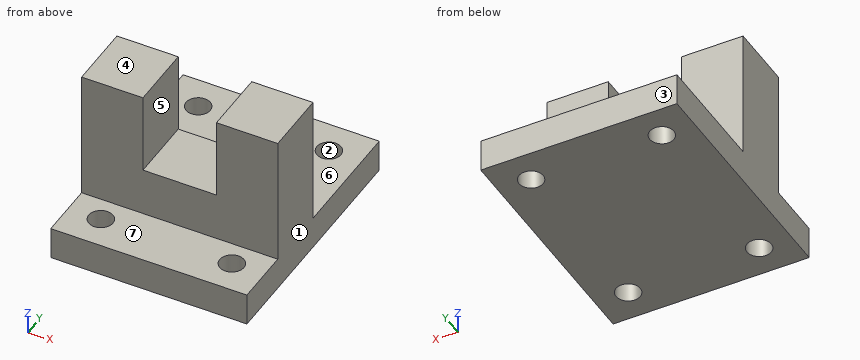
```python
from build123d import *

# Parameters (mm, degrees)
F0_W     = 23.8252
F0_H     = 31.75
F1_DEPTH = 25.4
F2_W     = 76.2
F2_H     = 12.7
F3_DEPTH = 47.625
F4_R     = 4.699
F5_DEPTH = 12.701
F6_R     = 4.699
F7_DEPTH = 33.02


with BuildPart() as f1:
    # F0 (on Front) → F1 (new body)
    with BuildSketch(Plane.XZ):
        with Locations((26.1874, 15.875)):
            Rectangle(F0_W, F0_H)
        Polygon((38.1, -31.75), (38.1, 0), (14.2748, 0), (-14.2748, 0), (-14.2748, 31.75), (-38.1, 31.75), (-38.1, -31.75), align=None)
    extrude(amount=F1_DEPTH)

    # F2 (on face) → F3 (join, symmetric)
    with BuildSketch(Plane(origin=(0, 0, 0), x_dir=(-1, 0, 0), z_dir=(0, 1, 0))):
        with Locations((0, -25.4)):
            Rectangle(F2_W, F2_H)
    extrude(amount=F3_DEPTH, both=True)

    # F4 (on face) → F5 (cut, through all)
    with BuildSketch(Plane.XY.offset(-19.05)):
        with Locations((-25.4996093811, -34.925)):
            Circle(F4_R)
        with Locations((25.4, -34.925)):
            Circle(F4_R)
    extrude(amount=-F5_DEPTH, mode=Mode.SUBTRACT)

    # F6 (on face) → F7 (cut, symmetric)
    with BuildSketch(Plane.XY.offset(-19.05)):
        with Locations((-25.4, 34.925)):
            Circle(F6_R)
        with Locations((25.4, 34.925)):
            Circle(F6_R)
    extrude(amount=F7_DEPTH, both=True, mode=Mode.SUBTRACT)


solid = f1.part
```
Verification items for the finished model (mm, model axes). Face numbers are marked on the shaded views. A direction names the side the tool comes from. Coordinates: 2 decimals unless noted, no trailing zeros. Loops run counter-clockwise (first coordinate to the right, second up) from the corner with the lowest first, then second, coordinate; pieces in that order, holes last. Notation, with made-up numbers: (-30, 22.5) -> (-21, 22.5) arc R24 ccw to (-21, 39.5) -> close; hole circle Ø4 at (-9, -16.5). An arc over 180 degrees is marked (long way). Put each result on its own line as item: value.
1. Section check D-D, the plane x = -4. Record the boundary of the cut face in (y, z) (3 decimals), then the cut area to 3 significant figures.
Result set:
outline: (-47.625, -31.75) -> (47.625, -31.75) -> (47.625, -19.05) -> (0, -19.05) -> (0, 0) -> (-25.4, 0) -> (-25.4, -19.05) -> (-47.625, -19.05) -> close
area: 1,690 mm^2
2. Section check B-B, the plane x = 25.4. Record the boundary of the cut face in (y, z) (3 decimals).
Result set:
outline: (-47.625, -31.75) -> (-39.624, -31.75) -> (-39.624, -19.05) -> (-47.625, -19.05) -> close; (-30.226, -31.75) -> (30.226, -31.75) -> (30.226, -19.05) -> (0, -19.05) -> (0, 31.75) -> (-25.4, 31.75) -> (-25.4, -19.05) -> (-30.226, -19.05) -> close; (39.624, -31.75) -> (47.625, -31.75) -> (47.625, -19.05) -> (39.624, -19.05) -> close
3. Gauge pin test, flat ends, axial feed: P1, Ø1.5, axis at x = -17, z = -7.5, coming from the -Y side; P2, Ø14.5, axis at x = -15, y = 32.5, coming from the +Z side; P3, Ø15, axis at x = 1.5, z = -5.5, coming from the +Y side. Record the tip position at first contact, or that the pin passes through.
Result set:
P1: stops at y = -25.4
P2: stops at z = -19.05
P3: stops at y = 0
4. Tool access check on the marked faces 4, 5, 6 and 7. Record the directions out of +Z, -Z, +X, -X, +Y, -Y that give a thin tool (end or side, any length) a straight path to the whole face; none if there is none.
Result set:
face 4: +Z, +X, -X, +Y, -Y
face 5: +Z, +Y, -Y
face 6: +Z, +X, -X, +Y
face 7: +Z, +X, -X, -Y
5. Section check C-C, the plane y = -16.5. Record the boundary of the cut face in (x, z).
Result set:
outline: (-38.1, -31.75) -> (38.1, -31.75) -> (38.1, 31.75) -> (14.27, 31.75) -> (14.27, 0) -> (-14.27, 0) -> (-14.27, 31.75) -> (-38.1, 31.75) -> close
6. Section check A-A, the plane z = 1.5. Record the boundary of the cut face in (x, y), then the cut area to 3 significant figures.
Result set:
outline: (-38.1, -25.4) -> (-14.27, -25.4) -> (-14.27, 0) -> (-38.1, 0) -> close; (14.27, -25.4) -> (38.1, -25.4) -> (38.1, 0) -> (14.27, 0) -> close
area: 1,210 mm^2
7. Mould release check, pull along X, two halves, no side actions. Record for the marked faces 1, 2 and 3: pulls with the +X half, pulls with the -X half, needs draft (parallel to the pull), parting line crosses it, or undercut.
Result set:
face 1: pulls with the +X half
face 2: undercut
face 3: needs draft
8. Thickness scan on line 1 (Y direction, x = -25.4, z = -22) (3 decimals); line 2 (X direction, y = 33.5, z = -20); line 3 (Z direction, x = -18, y = 24). Record the ranges inside material, lowest first.
Result set:
line 1: y = -47.625 to -39.623, -30.227 to 30.226, 39.624 to 47.625
line 2: x = -38.1 to -29.88, -20.92 to 20.92, 29.88 to 38.1
line 3: z = -31.75 to -19.05
